Answer from the drawing. Dimensions are ordinates in mm from the lowest x, y and z of the part. Round coordinates to 2 decimals unless told otherwise and drop trailing zeros. Order: outer loops, then holes, each group sorted by start corner. A loop starts at its lowest first (then second) coordinate and runs counter-clockwise, first axis right, second up.
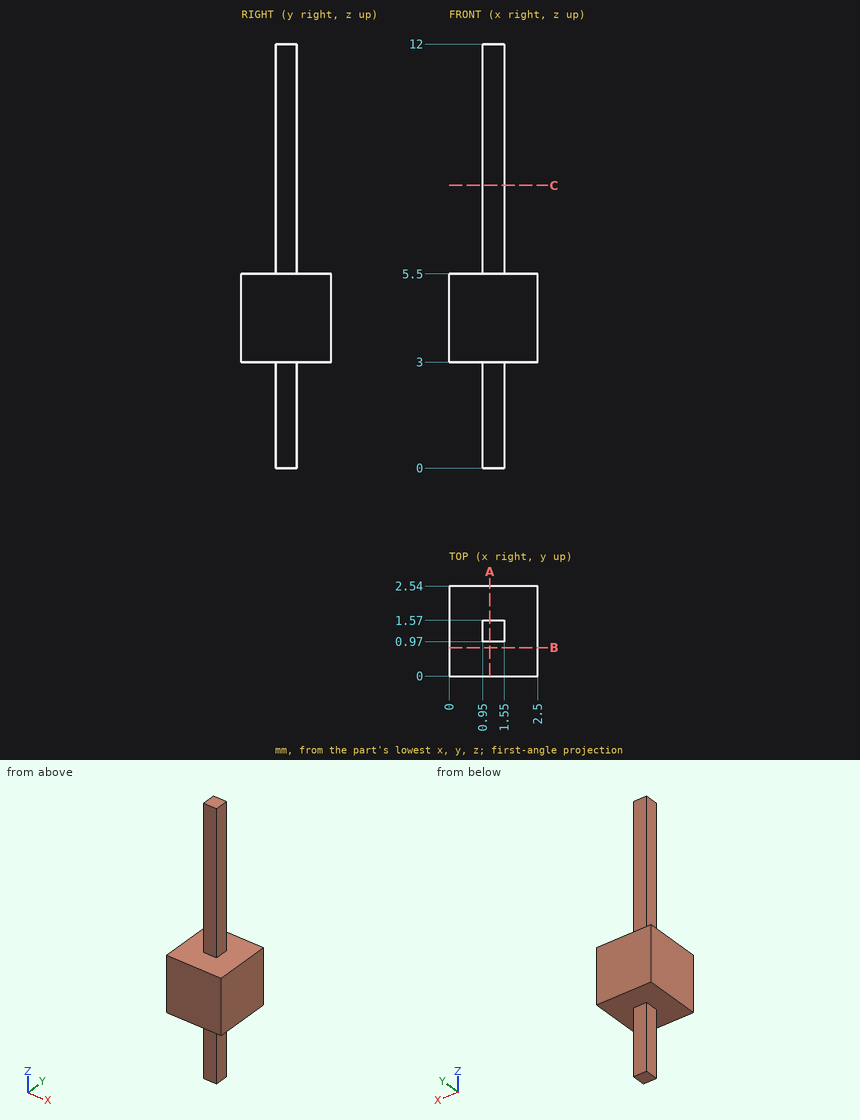
Q1. A cutting plane is placed at C-C, the plane z = 8. Give the vertices of the cut face in (x, y), plus the area to 3 significant figures.
Outcome:
outline: (0.95, 0.97) - (1.55, 0.97) - (1.55, 1.57) - (0.95, 1.57) - close
area: 0.360 mm2
Q2. Straight lines are drawn through the part: probe 1 along Z at (x, y) = (2.05, 0.45); probe 2 along Y at (x, z) = (1.15, 1.5); probe 3 along X at (y, z) = (1.45, 7). For each, find the intervals that lie inside material, in ascending order.
Outcome:
probe 1: z = 3 to 5.5
probe 2: y = 0.97 to 1.57
probe 3: x = 0.95 to 1.55
Q3. A cutting plane is placed at A-A, the plane x = 1.15. Give the vertices of the cut face in (y, z).
Outcome:
outline: (0, 3) - (0.97, 3) - (0.97, 0) - (1.57, 0) - (1.57, 3) - (2.54, 3) - (2.54, 5.5) - (1.57, 5.5) - (1.57, 12) - (0.97, 12) - (0.97, 5.5) - (0, 5.5) - close
Q4. A cutting plane is placed at B-B, the plane y = 0.8. Give the vertices of the cut face in (x, z).
Outcome:
outline: (0, 3) - (2.5, 3) - (2.5, 5.5) - (0, 5.5) - close
Q5. Flat-ended cylindrical pins translate along their axes: pin 1 (0.5 mm diameter, centred on y = 1.5, z = 9, fed in from +X); pin 2 (1 mm diameter, centred on y = 1, z = 6.5, fed in from -X); pin 3 (0.8 mm diameter, centred on x = 1, y = 2, fed in from +Z). Find the tip coordinate at first contact, or state that the pin passes through.
Outcome:
pin 1: stops at x = 1.55
pin 2: stops at x = 0.95
pin 3: stops at z = 5.5
